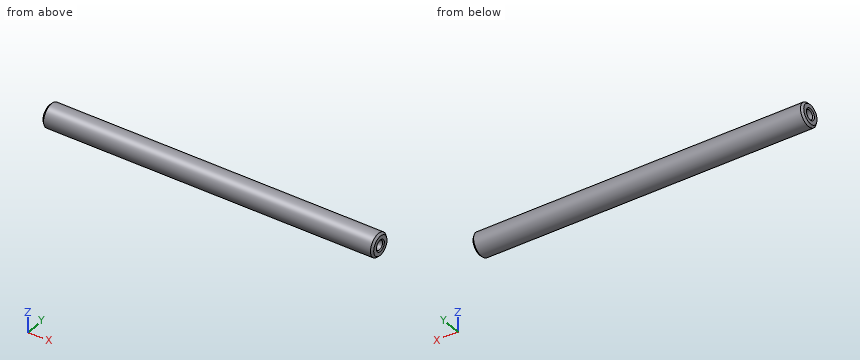
Autodesk Inventor part; units mm, degrees
ref_plane "YZ Plane" through (0, 0, 0) normal (1, 0, 0) x (0, 1, 0)
ref_plane "XZ Plane" through (0, 0, 0) normal (0, 1, 0) x (-1, 0, 0)
ref_plane "XY Plane" through (0, 0, 0) normal (0, 0, 1) x (1, 0, 0)
sketch "Sketch_1" plane through (0, 0, 0) normal (0, 0, 1) x (1, 0, 0)
  line L0 (86, 0) -> (0, 0)
  line L1 (0, 0) -> (0, 2.5)
  line L2 (0, 2.5) -> (0.5, 3)
  line L3 (0.5, 3) -> (85.5, 3)
  line L4 (85.5, 3) -> (86, 2.5)
  line L5 (86, 2.5) -> (86, 0)
  line L6 (86, 0) -> (0, 0)
revolve "Revolution1" add sketch "Sketch_1" angle 360 about axis through (86, 0, 0) along (1, 0, 0)
sketch "Sketch2" plane through (0, 0, 0) normal (-1, 0, 0) x (0, 0, 1)
  point P0 (0, 0)
hole "Hole1" at (0, 0, 0) direction (1, 0, 0) diameter 2.459 depth 6.7901 tip angle 120 countersink diameter 3 countersink angle 90
sketch "Sketch3" plane through (86, 0, 0) normal (1, 0, 0) x (0, 0, -1)
  point P0 (0, 0)
hole "Hole2" at (86, 0, 0) direction (-1, 0, 0) diameter 2.459 depth 6.7601 tip angle 120 countersink diameter 3 countersink angle 90
properties part number "RDOB6-86-WMC3"
Can you work these out from the model? Positions are in its coordinate system, mm. Coordinates: 2 decimals unless noted, no trailing zeros. Order: outer loops, then holes, each group sorted by start corner. A loop starts at its lowest first (then second) coordinate and runs counter-clockwise, first axis right, second up. Notation, with made-up numbers: (40.5, -35.5) - (56.5, -35.5) arc R18 cw to (56.5, -4.5) - close; hole circle Ø9 at (43.5, -19.5). An arc over 180 degrees is marked (long way). Answer in a Markdown table with one row per item.
1. Suppose I cut it at A-A (x = 13.5). Please give me the cut outline in (y, z), and give its area (3 significant figures).
Reply:
| item | result |
|---|---|
| outline | circle Ø6 at (0, 0) |
| area | 28.3 mm^2 |
2. If I drill on line 1 along Z through (x, y) = (4.75, 0); line 2 along Z through (x, y) = (22.5, 0.15), over which ranges is the centre line in solid material (lowest first)?
Reply:
| item | result |
|---|---|
| line 1 | z = -3 to -1.23, 1.23 to 3 |
| line 2 | z = -3 to 3 |
3. For pin 1 (1 mm diameter, centred on y = -0.5, z = -1, fed in from +X), with a flat end and sliding along its axis, tell me the tip position at first contact or that it passes through.
Reply:
| item | result |
|---|---|
| pin 1 | stops at x = 86 |
